Part print with two shaded views. Sizes in mm from the minimum x, y, z corner. A direction names the side the tool comes from. Give positions to 0.01 mm unless a question says otherwise; leave off trailing zeros. Write each loop counter-clockwise with the first axis right and the second up, starting at its lowest first coordinate (ties: lowest second). Pieces come first, ordered by that corner, then holes.
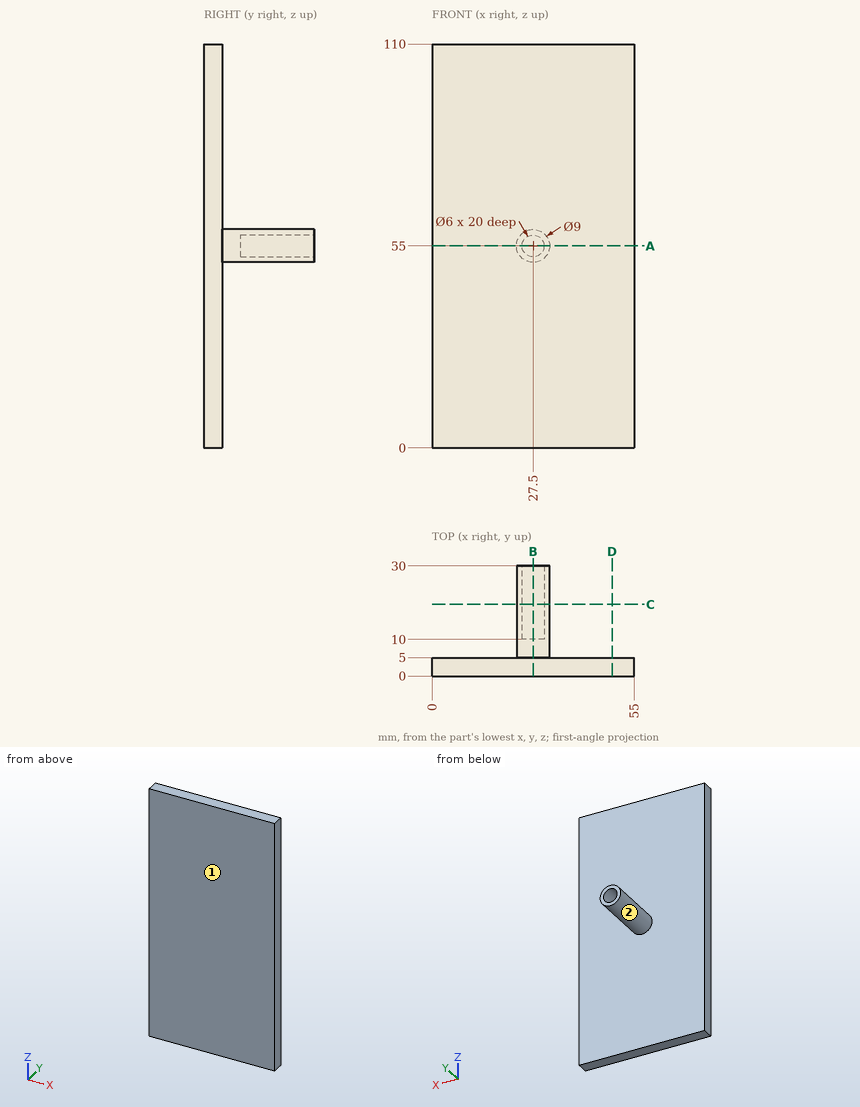
1) Saw through at A-A (z = 55). Write the cut outline in (x, y).
Check result:
outline: (0, 0) - (55, 0) - (55, 5) - (32, 5) - (32, 30) - (30.5, 30) - (30.5, 10) - (24.5, 10) - (24.5, 30) - (23, 30) - (23, 5) - (0, 5) - close
2) Saw through at B-B (x = 27.5). Write the cut outline in (y, z).
Check result:
outline: (0, 0) - (5, 0) - (5, 50.5) - (30, 50.5) - (30, 52) - (10, 52) - (10, 58) - (30, 58) - (30, 59.5) - (5, 59.5) - (5, 110) - (0, 110) - close
3) Flat gauge pins, fed straight in: P1, Ø5, axis at x = 26.5, z = 56, coming from the +Y side; P2, Ø8, axis at x = 13, z = 74.5, coming from the +Y side; P3, Ø8, axis at y = 14, z = 51, coming from the +X side. Where does each tip first touch, or does it go through?
Check result:
P1: stops at y = 30
P2: stops at y = 5
P3: stops at x = 32
4) 3-axis set-ups, long thin cutter, end or side, ignore diameter. For the marked faces 1 and 2: which of +Z, -Z, +X, -X, +Y, -Y reach the whole face in a straight line?
Check result:
face 1: +Z, -Z, +X, -X, -Y
face 2: +Y
5) Saw through at C-C (y = 19.5). Write the cut outline in (x, z), and give its area (3 significant figures).
Check result:
outline: circle Ø9 at (27.5, 55); hole circle Ø6 at (27.5, 55)
area: 35.3 mm2
6) Saw through at D-D (x = 49). Write the cut outline in (y, z).
Check result:
outline: (0, 0) - (5, 0) - (5, 110) - (0, 110) - close
7) Drill centre lines: L1, parallel to X at y = 16.5, z = 55; L2, parallel to Z at x = 27.5, y = 16.5; L3, parallel to Y at x = 9.5, z = 23. Where is each one in solid material? Low to high.
Check result:
L1: x = 23 to 24.5, 30.5 to 32
L2: z = 50.5 to 52, 58 to 59.5
L3: y = 0 to 5
